Check sheet for the modelled part. Datum: model origin and axes. Units: mm. A direction names the side the tool comes from. Coordinates: 2 decimals unless noted, no trailing zeros. Write each loop counter-clockwise with the first axis right and the second up, starting at its lowest first coordinate (ties: lowest second). Pieces come first, ordered by that corner, then holes. Notation, with made-up numbers: (27, -10.75) - (31, -10.75) arc R27 cw to (31, 25.25) - close; hole circle Ø8 at (56.5, 12). An arc over 180 degrees is marked (long way). Write each question's results on one line, items separated by ' | '.
from build123d import *

# Parameters (mm, degrees)
EXTRUDE_1_DEPTH        = 40
EXTRUDE_2_DEPTH        = 50
FILLET_1_R             = 15
CUT_EXTRUDE_1_DEPTH    = 50
FILLET_1_OF_MIRROR_2_R = 15
SKETCH_4_R             = 20
CUT_EXTRUDE_2_DEPTH    = 4.444444444
SKETCH_5_R             = 15.555555556
CUT_EXTRUDE_3_DEPTH    = 86.214294565
PATTERN_LINEAR_1_COUNT = 5
PATTERN_LINEAR_1_PITCH = 8.888888889


with BuildPart() as part:
    # 草图1 → 凸台-拉伸1 (new body)
    with BuildSketch(Plane(origin=(0, 0, 0), x_dir=(1, 0, 0), z_dir=(0, 1, 0))):
        with BuildLine():
            Line((-25, 0), (-12.5, -25))
            Line((-12.5, -25), (12.5, -25))
            Line((12.5, -25), (25, 0))
            ThreePointArc((25, 0), (0, 25), (-25, 0))
        make_face()
    extrude(amount=EXTRUDE_1_DEPTH)

    # 草图2 → 凸台-拉伸2 (add)
    with BuildSketch(Plane(origin=(20, 0, 10), x_dir=(0.447213595499958, 0, -0.894427190999916), z_dir=(0.894427190999916, 0, 0.447213595499958))):
        Polygon((8.180339887, 34), (8.180339887, 37), (-13.770509831, 37), (-13.770509831, 3), (8.180339887, 3), (8.180339887, 6), (-10.770509831, 6), (-10.770509831, 34), align=None)
    extrude_2 = extrude(amount=EXTRUDE_2_DEPTH)

    # 圆角1
    fillet_1_edges = [part.edges().sort_by_distance(p)[0] for p in [
        (68.379718763, 35.5, 25.043961348),
        (68.379718763, 4.5, 25.043961348),
    ]]
    fillet(fillet_1_edges, radius=FILLET_1_R)

    # 草图3 → 切除-拉伸1 (cut)
    with BuildSketch(Plane(origin=(-6.158359214, 0, 12.316718427), x_dir=(0.8944271909999159, 0, 0.44721359549995804), z_dir=(-0.44721359549995804, 0, 0.8944271909999159))):
        with BuildLine():
            Line((25.360679775, 26), (25.360679775, 14))
            ThreePointArc((25.360679775, 14), (27.703825526, 8.343145751), (33.360679775, 6))
            Line((33.360679775, 6), (61.360679775, 6))
            ThreePointArc((61.360679775, 6), (67.017534024, 8.343145751), (69.360679775, 14))
            Line((69.360679775, 14), (69.360679775, 26))
            ThreePointArc((69.360679775, 26), (67.017534024, 31.656854249), (61.360679775, 34))
            Line((61.360679775, 34), (33.360679775, 34))
            ThreePointArc((33.360679775, 34), (27.703825526, 31.656854249), (25.360679775, 26))
        make_face()
    cut_extrude_1 = extrude(amount=-CUT_EXTRUDE_1_DEPTH, mode=Mode.SUBTRACT)

    # 镜向2: 凸台-拉伸2, 切除-拉伸1 across plane
    add(extrude_2.mirror(Plane(origin=(0, 0, 0), x_dir=(0, 0, 1), z_dir=(1, 0, 0))))
    add(cut_extrude_1.mirror(Plane(origin=(0, 0, 0), x_dir=(0, 0, 1), z_dir=(1, 0, 0))), mode=Mode.SUBTRACT)

    # 圆角1 of 镜向2
    fillet_1_of_mirror_2_edges = [part.edges().sort_by_distance(p)[0] for p in [
        (-68.379718763, 35.5, 25.043961348),
        (-68.379718763, 4.5, 25.043961348),
    ]]
    fillet(fillet_1_of_mirror_2_edges, radius=FILLET_1_OF_MIRROR_2_R)

    # 草图4 → 切除-拉伸2 (cut)
    with BuildSketch(Plane(origin=(0, 40, 0), x_dir=(1, 0, 0), z_dir=(0, 1, 0))):
        with Locations(Location((0, 0, 0), (0, 0, 270))):
            Circle(SKETCH_4_R)
    cut_extrude_2 = extrude(amount=-CUT_EXTRUDE_2_DEPTH, mode=Mode.SUBTRACT)

    # 草图5 → 切除-拉伸3 (cut, through all)
    with BuildSketch(Plane(origin=(0, 35.555555556, 0), x_dir=(1, 0, 0), z_dir=(0, 1, 0))):
        with Locations(Location((0, 0, 0), (0, 0, 270))):
            Circle(SKETCH_5_R)
    extrude(amount=-CUT_EXTRUDE_3_DEPTH, mode=Mode.SUBTRACT)

    # 阵列(线性)1: 切除-拉伸2 ×5
    with Locations(*[(0, -i * PATTERN_LINEAR_1_PITCH, 0) for i in range(1, PATTERN_LINEAR_1_COUNT)]):
        add(cut_extrude_2, mode=Mode.SUBTRACT)


solid = part.part
1. Draft check along Z on faces 4 (the flat face through (-41, 37, 23)), 5 (the flat face through (-17.186, 20.084, 22.336)), 6 (the cylindrical face through (-19.524, 28.92, -4.336)), 7 (the cylindrical face through (62.43, 4.52, 26.85)). Enter one of: pulls with the +Z half, pulls with the -Z half, needs draft (parallel to the pull), parting line crosses it, or undercut.
Values follow:
face 4: needs draft | face 5: pulls with the +Z half | face 6: undercut | face 7: parting line crosses it
2. Sectioned sample at C-C (y = 11). Record the cut outline in (x, z), then the cut area to 3 significant figures.
Values follow:
outline: (-59.9, 41.99) - (-56.7, 40.39) - (-55.36, 43.07) - (-58.56, 44.68) - close; (-25, 0) arc R25 ccw to (25, 0) - (15.18, 19.63) - (18.39, 21.24) - (17.05, 23.92) - (13.84, 22.32) - (12.5, 25) - (-12.5, 25) - (-13.84, 22.32) - (-17.05, 23.92) - (-18.39, 21.24) - (-15.18, 19.63) - close; (55.36, 43.07) - (56.7, 40.39) - (59.9, 41.99) - (58.56, 44.68) - close; hole circle Ø40 at (0, 0) | area: 706 mm^2
3. Sectioned sample at B-B (x = -42). Record the cut outline in (y, z), then the cut area to 3 significant figures.
Values follow:
outline: (3, 11.85) - (6, 11.85) - (6, 36.4) - (3, 36.4) - close; (34, 11.85) - (37, 11.85) - (37, 36.4) - (34, 36.4) - close | area: 147 mm^2
4. Material ranges on L1, parallel to X at y = 20.9, z = 0; L2, parallel to Y at x = 28, z = 10; L3, parallel to X at y = 34, z = 0, recorded low to high. Write a range as [from, to].
Values follow:
L1: x = [-25, -20], [20, 25] | L2: y = [3, 6], [34, 37] | L3: x = [-25, -15.56], [15.56, 25]
5. Go/stop test with flat-tipped pins: pin 1 (4 mm diameter, centred on x = 36, z = 23, fed in from +Y); pin 2 (12 mm diameter, centred on x = -19.5, z = 21, fed in from +Y); pin 3 (8 mm diameter, centred on y = 11, z = -0.5, fed in from +X); pin 4 (6 mm diameter, centred on y = 35, z = 17.5, fed in from +X). Record where each tip stops, or that it passes through.
Values follow:
pin 1: stops at y = 37 | pin 2: stops at y = 40 | pin 3: stops at x = 25 | pin 4: stops at x = 58.17
6. Sectioned sample at A-A (y = 21). Record the cut outline in (x, z), then the cut area to 3 significant figures.
Values follow:
outline: (-59.9, 41.99) - (-57.22, 40.65) - (-55.88, 43.34) - (-58.56, 44.68) - close; (-25, 0) arc R25 ccw to (25, 0) - (15.18, 19.63) - (17.87, 20.98) - (16.52, 23.66) - (13.84, 22.32) - (12.5, 25) - (-12.5, 25) - (-13.84, 22.32) - (-16.52, 23.66) - (-17.87, 20.98) - (-15.18, 19.63) - close; (55.88, 43.34) - (57.22, 40.65) - (59.9, 41.99) - (58.56, 44.68) - close; hole circle Ø40 at (0, 0) | area: 699 mm^2
7. Access from +Z, -Z, +X, -X, +Y, -Y to the whole of each face (thin tool, end or side, straight path). Record for faces 1 (the flat face through (57.88, 19.93, 40.98)), 2 (the flat face through (-10.3, 31.111, -11.9)), 3 (the flat face through (17.186, 20.084, 22.336)).
Values follow:
face 1: -Z, +X | face 2: none | face 3: +Z, +X
